Build history of the part. All positions in model axes, mm. A direction names the side the tool comes from. Give positions to 0.01 mm unless a question says otherwise; leave off trailing zeros. Loops run counter-clockwise (first coordinate to the right, second up) from the corner with the lowest first, then second, coordinate; pieces in that order, holes last. Notation, with made-up numbers: (60.25, -39) -> (104.25, -39) arc R23 cw to (104.25, -17) -> close; hole circle Ø6 at (-18.5, 48). An arc over 180 degrees is marked (long way). One line per question, with ' | ' between items. Start each with the question number.
(1) 3-axis set-ups, long thin cutter, end or side, ignore diameter. For faces 5 (the face through (-19, 2, -1.4)), 6 (the face through (-19, 1, 6)), 7 (the face through (19, 2, -1.4)), 8 (the face through (11.5, 7, 3)), 9 (the face through (-14, 7, -8.375)): which of +Z, -Z, +X, -X, +Y, -Y reach the whole face in a straight line?
(2) Slice it at C-C, the plane x = -19. Write the cut outline in (y, z).
(3) Slice it at D-D, the plane z = -11.75. Write the cut outline in (x, y).
(4) Mould opens along Z. For faces 1 (the face through (19, 1, 6)), 2 (the face through (20, 1, 0)), 3 (the face through (-14, 7, -5.2)), 4 (the face through (-14, 13, 2)) say: pulls with the +Z half, pulls with the -Z half, needs draft (parallel to the pull), parting line crosses it, or undercut.
(5) Slice it at A-A, the plane y = 11.75. Write the cut outline in (x, z) (3 decimals), then the cut area to 3 significant figures.
(6) Flat gauge pins, fed straight in: pin 1 Ø2 at (y, z) = (7.5, -1.5) entering from +X; pin 2 Ø6 at (y, z) = (9, 0.5) entering from -X; pin 3 Ø14 at (x, z) = (4, -1.5) entering from +Y. Where does each tip first touch, or does it go through?
(7) Slice it at B-B, the plane z = 0. Write the cut outline in (x, y), then the cut area to 3 significant figures.
(8) Drill centre lines: L1, parallel to X at y = 1.25, z = 0; L2, parallel to X at y = 0.55, z = 0; L3, parallel to Z at x = 19, y = 1. Where is each one in solid material? Low to high. Write a range as from..to.
```python
from build123d import *

# Parameters (mm, degrees)
SKETCH1_W           = 31
SKETCH1_H           = 28.4
BOSS_EXTRUDE1_DEPTH = 1
SKETCH3_W           = 4
SKETCH3_H           = 19.4
SKETCH3_H_2         = 5.825
SKETCH3_H_3         = 5.82
BOSS_EXTRUDE2_DEPTH = 12
SKETCH4_W           = 31
SKETCH4_H           = 4
CUT_EXTRUDE1_DEPTH  = 12
SKETCH7_W           = 7
SKETCH7_H           = 12
BOSS_EXTRUDE3_DEPTH = 2
SKETCH8_R           = 1
CUT_EXTRUDE4_DEPTH  = 29.790449805


with BuildPart() as part:
    # Sketch1 → Boss-Extrude1 (new body)
    with BuildSketch(Plane(origin=(0, 0, 0), x_dir=(1, 0, 0), z_dir=(0, 1, 0))):
        Rectangle(SKETCH1_W, SKETCH1_H)
    extrude(amount=BOSS_EXTRUDE1_DEPTH)

    # Sketch3 → Boss-Extrude2 (add)
    with BuildSketch(Plane(origin=(0, 1, 0), x_dir=(1, 0, 0), z_dir=(0, 1, 0))):
        with Locations((-13.5, -4.5)):
            Rectangle(SKETCH3_W, SKETCH3_H)
        with Locations((13.5, -4.5)):
            Rectangle(SKETCH3_W, SKETCH3_H)
        with Locations((-13.5, 11.2875)):
            Rectangle(SKETCH3_W, SKETCH3_H_2)
        with Locations((13.5, 11.29)):
            Rectangle(SKETCH3_W, SKETCH3_H_3)
    extrude(amount=BOSS_EXTRUDE2_DEPTH)

    # Sketch4 → Cut-Extrude1 (cut)
    with BuildSketch(Plane(origin=(0, 13, 0), x_dir=(1, 0, 0), z_dir=(0, 1, 0))):
        with Locations((0, -12.2)):
            Rectangle(SKETCH4_W, SKETCH4_H)
    extrude(amount=-CUT_EXTRUDE1_DEPTH, mode=Mode.SUBTRACT)

    # Sketch7 → Boss-Extrude3 (add)
    with BuildSketch(Plane(origin=(0, 0, 0), x_dir=(1, 0, 0), z_dir=(0, 1, 0))):
        with Locations((19, 0)):
            Rectangle(SKETCH7_W, SKETCH7_H)
        with Locations((-19, 0)):
            Rectangle(SKETCH7_W, SKETCH7_H)
    extrude(amount=BOSS_EXTRUDE3_DEPTH)

    # Sketch8 → Cut-Extrude4 (cut, through all)
    with BuildSketch(Plane(origin=(0, 2, 0), x_dir=(1, 0, 0), z_dir=(0, 1, 0))):
        with Locations(Location((-19, 0, 0), (0, 0, 270))):
            Circle(SKETCH8_R)
        with Locations(Location((19, 0, 0), (0, 0, 90))):
            Circle(SKETCH8_R)
    extrude(amount=-CUT_EXTRUDE4_DEPTH, mode=Mode.SUBTRACT)


solid = part.part
```
Final values:
1) face 5: +Z, -Z, -X, +Y | face 6: +Z, -X, +Y, -Y | face 7: +Z, -Z, +X, +Y | face 8: +Z, -Z, +Y | face 9: +X, -X, +Y
2) outline: (0, -6) -> (2, -6) -> (2, -1) -> (0, -1) -> close; (0, 1) -> (2, 1) -> (2, 6) -> (0, 6) -> close
3) outline: (-15.5, 0) -> (15.5, 0) -> (15.5, 13) -> (11.5, 13) -> (11.5, 1) -> (-11.5, 1) -> (-11.5, 13) -> (-15.5, 13) -> close
4) face 1: pulls with the +Z half | face 2: undercut | face 3: undercut | face 4: needs draft
5) outline: (-15.5, -14.2) -> (-11.5, -14.2) -> (-11.5, -8.375) -> (-15.5, -8.375) -> close; (-15.5, -5.2) -> (-11.5, -5.2) -> (-11.5, 10.2) -> (-15.5, 10.2) -> close; (11.5, -14.2) -> (15.5, -14.2) -> (15.5, -8.38) -> (11.5, -8.38) -> close; (11.5, -5.2) -> (15.5, -5.2) -> (15.5, 10.2) -> (11.5, 10.2) -> close | area: 170 mm2
6) pin 1: x = 15.5 | pin 2: x = -15.5 | pin 3: y = 1
7) outline: (-22.5, 0) -> (-20, 0) -> (-20, 2) -> (-22.5, 2) -> close; (-18, 0) -> (18, 0) -> (18, 2) -> (15.5, 2) -> (15.5, 13) -> (11.5, 13) -> (11.5, 1) -> (-11.5, 1) -> (-11.5, 13) -> (-15.5, 13) -> (-15.5, 2) -> (-18, 2) -> close; (20, 0) -> (22.5, 0) -> (22.5, 2) -> (20, 2) -> close | area: 147 mm2
8) L1: -22.5..-20, -18..-11.5, 11.5..18, 20..22.5 | L2: -22.5..-20, -18..18, 20..22.5 | L3: -6..-1, 1..6
